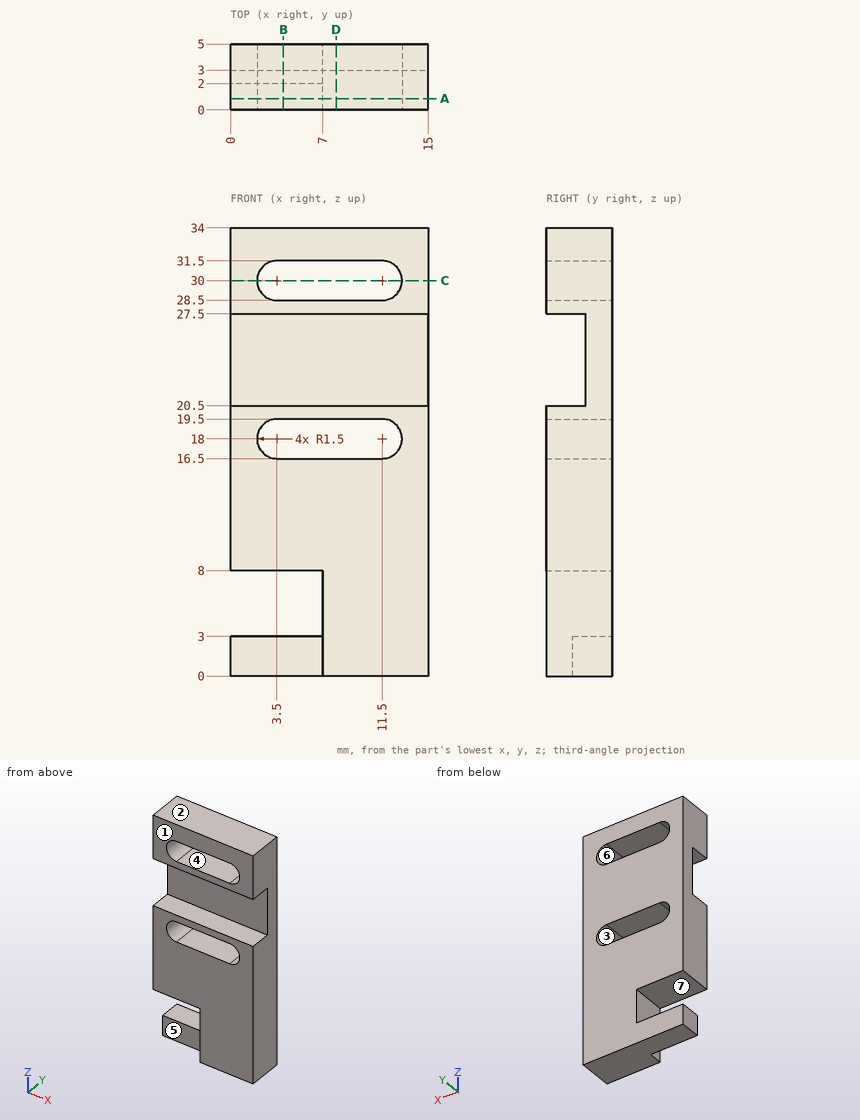
Can you work these out from the drawing? Everything is in mm from the part's minimum corner. A direction names the side the tool comes from. Coordinates: 2 decimals unless noted, no trailing zeros. Loops run counter-clockwise (first coordinate to the right, second up) from the corner with the lowest first, then second, coordinate; pieces in that order, holes last. Notation, with made-up numbers: M 56.25,-30.5 L 91.25,-30.5 A27 ccw 91.25,-12.5 Z; hole C 58.25,68.5 d5. An arc over 180 degrees is marked long. One line per item, written item: value.
1. Imagine slicing it at B-B (x = 4). List the corners of the cut face in (y, z) for me, and give its area (3 significant figures).
Geometry says:
outline: M 0,8 L 5,8 L 5,16.5 L 0,16.5 Z; M 0,19.5 L 5,19.5 L 5,28.5 L 0,28.5 L 0,27.5 L 3,27.5 L 3,20.5 L 0,20.5 Z; M 0,31.5 L 5,31.5 L 5,34 L 0,34 Z; M 2,0 L 5,0 L 5,3 L 2,3 Z
area: 88.0 mm2
2. On a 3-axis mill with a long thin cutter (end or side, diameter ignored), from which of +Z, -Z, +X, -X, +Y, -Y can I reach the whole of each face in a straight line? I mean the marked faces 5, 6 and 7. Say none if no direction works.
Geometry says:
face 5: -Z, -X, -Y
face 6: +Y, -Y
face 7: -X, +Y, -Y
3. Thinking about a two-plate mould opening in Z: for the marked faces 1, 2, 3 and 4, which applies, +Z half, -Z half, draft (parallel to the pull), parting line (faces both ways), or undercut?
Geometry says:
face 1: draft
face 2: +Z half
face 3: undercut
face 4: undercut
4. Will these pins go through, and if not, where does the flat tip stop? pin 1 Ø3.5 at (x, z) = (5, 2) entering from -Y; pin 2 Ø3.5 at (x, z) = (5.5, 24.5) entering from -Y.
Geometry says:
pin 1: stops at y = 2
pin 2: stops at y = 3
5. Please list where these lines run through material, in increasing order: probe 1 along Z at (x, y) = (7.25, 4.6); probe 2 along Z at (x, y) = (8.5, 2.7); probe 3 along Z at (x, y) = (6.5, 4.7).
Geometry says:
probe 1: z = 0 to 16.5, 19.5 to 28.5, 31.5 to 34
probe 2: z = 0 to 16.5, 19.5 to 20.5, 27.5 to 28.5, 31.5 to 34
probe 3: z = 0 to 3, 8 to 16.5, 19.5 to 28.5, 31.5 to 34
6. Imagine slicing it at D-D (x = 8). List the corners of the cut face in (y, z) for me.
Geometry says:
outline: M 0,0 L 5,0 L 5,16.5 L 0,16.5 Z; M 0,19.5 L 5,19.5 L 5,28.5 L 0,28.5 L 0,27.5 L 3,27.5 L 3,20.5 L 0,20.5 Z; M 0,31.5 L 5,31.5 L 5,34 L 0,34 Z
7. Imagine slicing it at C-C (z = 30). List the corners of the cut face in (x, y) for me, and give its area (3 significant figures).
Geometry says:
outline: M 0,0 L 2,0 L 2,5 L 0,5 Z; M 13,0 L 15,0 L 15,5 L 13,5 Z
area: 20.0 mm2
8. Imagine slicing it at A-A (y = 0.85). List the corners of the cut face in (x, z) for me.
Geometry says:
outline: M 0,8 L 7,8 L 7,0 L 15,0 L 15,20.5 L 0,20.5 Z; M 0,27.5 L 15,27.5 L 15,34 L 0,34 Z; hole M 3.5,16.5 L 11.5,16.5 A1.5 ccw 11.5,19.5 L 3.5,19.5 A1.5 ccw Z; hole M 3.5,28.5 L 11.5,28.5 A1.5 ccw 11.5,31.5 L 3.5,31.5 A1.5 ccw Z
